Could you check a few things on this drawing? It's one solid part, dimensions in mm from its lowest x, y, z. Give positions to 0.01 mm unless a question says otherwise; leave off trailing zeros. Loops run counter-clockwise (first coordinate to the right, second up) from the corner with the lowest first, then second, coordinate; pieces in that order, holes last. Notation, with made-up numbers: M -25,64 L -5,64 A20 ccw -5,85 Z; hole C -20,48 d2. An arc over 180 degrees is marked long. Answer as a JSON object with one key per item and string values.
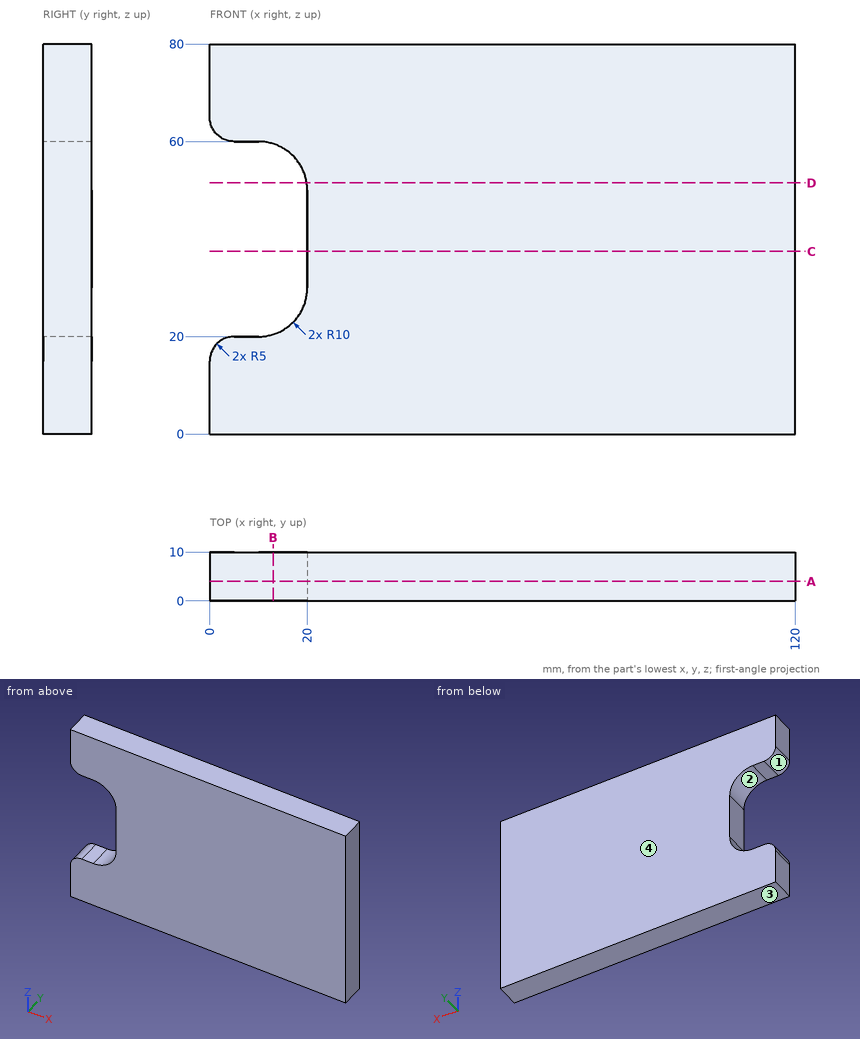
1) Suppose I cut it at A-A, the plane y = 4. Write out the boundary of the cut face in (x, z).
Answer list:
{"outline": "M 0,0 L 120,0 L 120,80 L 0,80 L 0,65 A5 ccw 5,60 L 10,60 A10 cw 20,50 L 20,30 A10 cw 10,20 L 5,20 A5 ccw 0,15 Z"}
2) Suppose I cut it at D-D, the plane z = 51.5. Write out the boundary of the cut face in (x, y), and give its area (3 significant figures).
Answer list:
{"outline": "M 19.89,0 L 120,0 L 120,10 L 19.89,10 Z", "area": "1,000 mm^2"}
3) Please list where these lines run through material, in increasing order: line 1 along X through (y, z) = (6.25, 46.5); line 2 along Z through (x, y) = (15, 1.5); line 3 along Z through (x, y) = (19, 1). Write a range as from..to.
Answer list:
{"line 1": "20..120", "line 2": "0..21.34, 58.66..80", "line 3": "0..25.64, 54.36..80"}
4) If we mould it in two halves opening along Z, with no side actions, what happens to the marked faces 1, 2, 3 and 4? For each: +Z half, -Z half, draft (parallel to the pull), parting line (faces both ways), or undercut.
Answer list:
{"face 1": "undercut", "face 2": "undercut", "face 3": "-Z half", "face 4": "draft"}
5) Suppose I cut it at B-B, the plane x = 13. Write out the boundary of the cut face in (y, z), and give its area (3 significant figures).
Answer list:
{"outline": "M 0,0 L 10,0 L 10,20.46 L 0,20.46 Z; M 0,59.54 L 10,59.54 L 10,80 L 0,80 Z", "area": "409 mm^2"}
6) Suppose I cut it at C-C, the plane z = 37.5. Write out the boundary of the cut face in (x, y).
Answer list:
{"outline": "M 20,0 L 120,0 L 120,10 L 20,10 Z"}
